The drawing under review shows one solid part. Ordinate dimensions are in mm from its lowest x, y, z. Give positions to 0.01 mm unless a question says otherwise; leave off trailing zeros. Loops run counter-clockwise (first coordinate to the right, second up) from the corner with the lowest first, then second, coordinate; pieces in that order, holes last. Notation, with made-up numbers: (-23.75, 85.25) - (24.25, 85.25) arc R9 cw to (24.25, 100.25) - close; hole circle Ø7 at (81.5, -23). An arc over 180 degrees is marked (long way). Put each result on its own line as item: value. Start each with the question number.
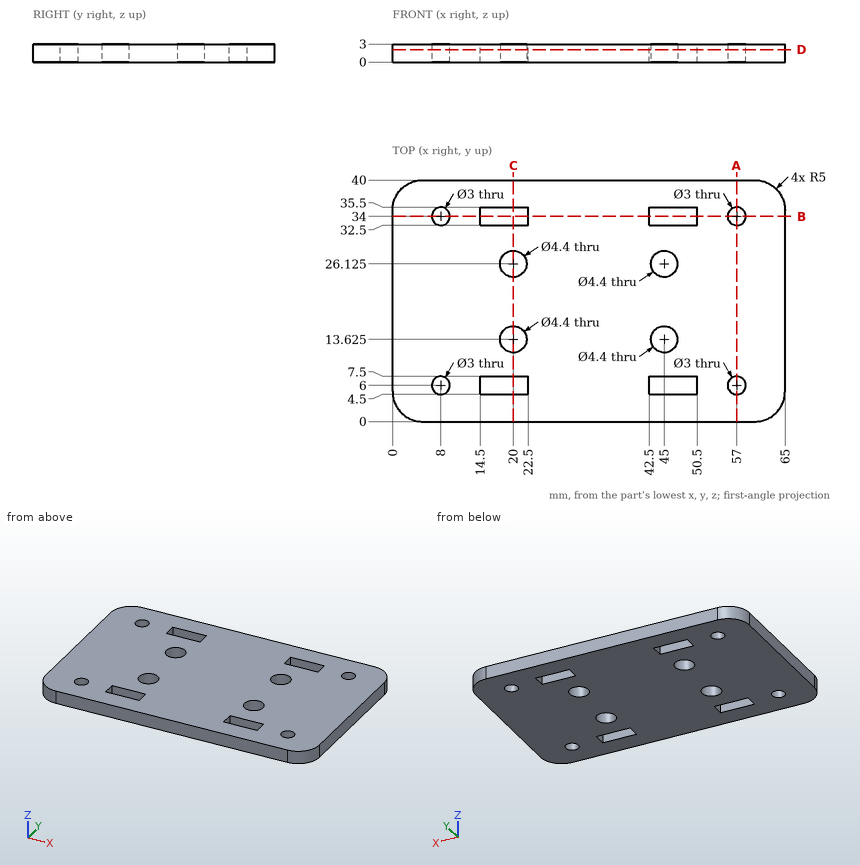
Item 1: Consider section C-C (x = 20). State the section outline as (y, z) points (3 decimals).
Item 2: For L1, parallel to Y at x = 20, z = 1.2 (3 decimals); L2, parallel to Y at x = 58, z = 0.85; L3, parallel to X at y = 35, z = 0.2, list the stretches that pass through material, from the lowest coordinate up. Write a range as from..to.
Item 3: Consider section B-B (y = 34). State the section outline as (x, z) points.
Item 4: Consider section D-D (z = 2.05). Count the separate pieces of the cut face and the enclosed holes in it, plus the area to 3 significant figures.
Item 5: Consider section A-A (x = 57). State the section outline as (y, z) points.
Geometry says:
1. outline: (0, 0) - (4.5, 0) - (4.5, 3) - (0, 3) - close; (7.5, 0) - (11.425, 0) - (11.425, 3) - (7.5, 3) - close; (15.825, 0) - (23.925, 0) - (23.925, 3) - (15.825, 3) - close; (28.325, 0) - (32.5, 0) - (32.5, 3) - (28.325, 3) - close; (35.5, 0) - (40, 0) - (40, 3) - (35.5, 3) - close
2. L1: y = 0..4.5, 7.5..11.425, 15.825..23.925, 28.325..32.5, 35.5..40
2. L2: y = 0..4.88, 7.12..32.88, 35.12..40
2. L3: x = 0..6.88, 9.12..14.5, 22.5..42.5, 50.5..55.88, 58.12..65
3. outline: (0, 0) - (6.5, 0) - (6.5, 3) - (0, 3) - close; (9.5, 0) - (14.5, 0) - (14.5, 3) - (9.5, 3) - close; (22.5, 0) - (42.5, 0) - (42.5, 3) - (22.5, 3) - close; (50.5, 0) - (55.5, 0) - (55.5, 3) - (50.5, 3) - close; (58.5, 0) - (65, 0) - (65, 3) - (58.5, 3) - close
4. separate pieces: 1
4. enclosed holes: 12
4. area: 2,390 mm2
5. outline: (0, 0) - (4.5, 0) - (4.5, 3) - (0, 3) - close; (7.5, 0) - (32.5, 0) - (32.5, 3) - (7.5, 3) - close; (35.5, 0) - (40, 0) - (40, 3) - (35.5, 3) - close
